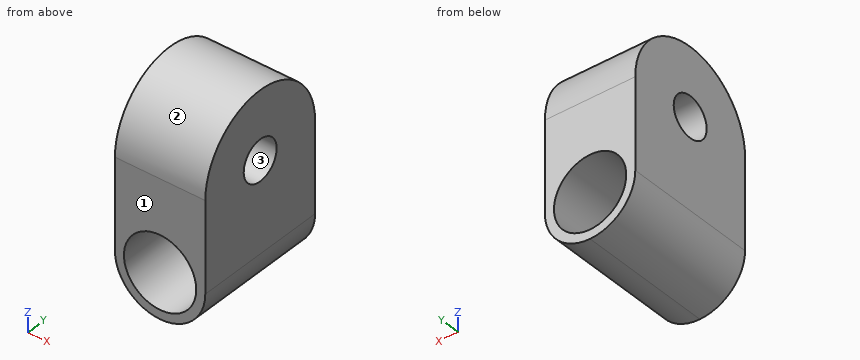
from build123d import *

# Parameters (mm, degrees)
SKETCH1_R               = 2.25
BOSS_EXTRUDE1_DEPTH     = 5
SKETCH2_R               = 4
CUT_EXTRUDE1_DEPTH      = 1
CUT_EXTRUDE1_DEPTH_BACK = 16


with BuildPart() as part:
    # Sketch1 → Boss-Extrude1 (new body, symmetric)
    with BuildSketch(Plane(origin=(0, 0, 0), x_dir=(0, 0, -1), z_dir=(1, 0, 0))):
        with BuildLine():
            Line((7.5, -7.5), (-7.5, -7.5))
            ThreePointArc((-7.5, -7.5), (-15, 0), (-7.5, 7.5))
            Line((-7.5, 7.5), (7.5, 7.5))
            Line((7.5, 7.5), (7.5, -7.5))
        make_face()
        with Locations((-7.5, 0)):
            Circle(SKETCH1_R, mode=Mode.SUBTRACT)
    extrude(amount=BOSS_EXTRUDE1_DEPTH, both=True)

    # Sketch2 → Cut-Extrude1 (cut, two sides)
    with BuildSketch(Plane(origin=(0, 7.5, 0), x_dir=(1, 0, 0), z_dir=(0, 1, 0))) as cut_extrude1_sk:
        Polygon((-5, 10.919306059), (-5, 7.5), (0, 7.5), (5, 7.5), (5, 10.919306059), align=None)
        with BuildLine():
            Line((-5, 7.5), (-5, 2.5))
            ThreePointArc((-5, 2.5), (-3.535533906, 6.035533906), (0, 7.5))
            Line((0, 7.5), (-5, 7.5))
        make_face()
        with BuildLine():
            ThreePointArc((0, 7.5), (3.535533906, 6.035533906), (5, 2.5))
            Line((5, 2.5), (5, 7.5))
            Line((5, 7.5), (0, 7.5))
        make_face()
        with Locations((0, 2.5)):
            Circle(SKETCH2_R)
    extrude(amount=CUT_EXTRUDE1_DEPTH, mode=Mode.SUBTRACT)
    extrude(cut_extrude1_sk.sketch, amount=-CUT_EXTRUDE1_DEPTH_BACK, mode=Mode.SUBTRACT)


solid = part.part
Source: CAD feature listing. Evaluate the final solid. Frame: model axes, mm. Face numbers are marked on the shaded views. Round coordinates to 2 decimals unless told otherwise and drop trailing zeros. Write each loop counter-clockwise with the first axis right and the second up, starting at its lowest first coordinate (ties: lowest second). Pieces come first, ordered by that corner, then holes. Notation, with made-up numbers: (35.5, 30) - (72.5, 30) arc R16 cw to (72.5, 50) - close; hole circle Ø7 at (47.25, 60.5). An arc over 180 degrees is marked (long way). Use CSV: the item, a comma, the result in double quotes. Start each with the question number.
(1) Material intervals for probe 1 along Z at (x, y) = (-1.25, -0.75); probe 2 along X at (y, z) = (-4, -2.5); probe 3 along Y at (x, z) = (-0.25, 7.5), sorted ascending. Write a range as [from, to].
(2) Cut plane B-B, the plane x = 1. Return loops of the section in (y, z).
(3) Mould query, pull axis Z, two halves, no side actions, for the marked faces 1, 2 and 3. Classes: pulls with the +Z half, pulls with the -Z half, needs draft (parallel to the pull), parting line crosses it, or undercut.
(4) First-contact query: pin 1 Ø2 at (x, y) = (2.5, -3) entering from -Z; pin 2 Ø2 at (x, y) = (-3, 3.5) entering from +Z; pin 3 Ø1.5 at (x, y) = (-4, -2.5) entering from +Z. Flat tips, straight axial feed; report the tip coordinate or a pass-through.
(5) Cut plane C-C, the plane z = 6.25. Return loops of the section in (x, y), and give its area (3 significant figures).
(6) Cut plane D-D, the plane x = 3. Return loops of the section in (y, z).
(7) Cut plane A-A, the plane y = 0. Return loops of the section in (x, z).
Geometry says:
1,probe 1,"[-7.34, -6.3], [1.3, 5.38], [9.62, 14.96]"
1,probe 2,"[-5, -4], [4, 5]"
1,probe 3,"[-7.5, -2.25], [2.25, 7.5]"
2,outline,"(-7.5, -7.4) - (7.5, -7.4) - (7.5, -6.37) - (-7.5, -6.37) - close; (-7.5, 1.37) - (7.5, 1.37) - (7.5, 7.5) arc R7.5 ccw to (-7.5, 7.5) - close; hole circle Ø4.5 at (0, 7.5)"
3,face 1,"needs draft"
3,face 2,"pulls with the +Z half"
3,face 3,"undercut"
4,pin 1,"z = -7.27"
4,pin 2,"z = 14.57"
4,pin 3,"z = 14.79"
5,outline,"(-5, -7.5) - (5, -7.5) - (5, -1.87) - (-5, -1.87) - close; (-5, 1.87) - (5, 1.87) - (5, 7.5) - (-5, 7.5) - close"
5,area,"113 mm²"
6,outline,"(-7.5, -6.5) - (7.5, -6.5) - (7.5, -5.15) - (-7.5, -5.15) - close; (-7.5, 0.15) - (7.5, 0.15) - (7.5, 7.5) arc R7.5 ccw to (-7.5, 7.5) - close; hole circle Ø4.5 at (0, 7.5)"
7,outline,"(-5, -2.5) arc R5 ccw to (5, -2.5) - (5, 5.25) - (-5, 5.25) - close; (-5, 9.75) - (5, 9.75) - (5, 15) - (-5, 15) - close; hole circle Ø8 at (0, -2.5)"
